Input: part model. Units: mm. Frame: model coordinates. Round coordinates to 2 decimals unless told otherwise and drop trailing zeros. Loops run counter-clockwise (first coordinate to the right, second up) from the corner with the lowest first, then second, coordinate; pieces in that order, holes last. Notation, with made-up numbers: M 66.25,-30 L 112.25,-30 A21 cw 112.25,-24 Z; hole C 35.25,19 d8. An arc over 180 degrees is marked long. Use one line per item in the form item = value. Start each with the question number.
Q1. Section query D-D, the plane x = 173. Output: boundary loops of the cut face in (y, z), and give its area (3 significant figures).
Q2. First-contact query: P1, Ø2, axis at x = 38, y = 2, coming from the -Z side; P2, Ø1.5, axis at x = 132.5, y = 3.5, coming from the +Z side; P3, Ø2.5, axis at y = 2.5, z = -45, coming from the -X side. Flat tips, straight axial feed; report the tip coordinate or a pass-through.
Q3. Section query A-A, the plane x = 25. Output: boundary loops of the cut face in (y, z), and give its area (3 significant figures).
Q4. Ray query, line 1 along X through (y, z) = (0.7, 62.5); line 2 along Z through (x, y) = (108, 2.55); line 3 along Z through (x, y) = (184, 3.8). Return the intervals inside material, ascending.
Q5. Section query B-B, the plane y = 2.2. State how many separate pieces and enclosed holes the cut face has, and give its area (3 significant figures).
Q6. Section query C-C, the plane z = 153. Output: boundary loops of the cut face in (x, y).
```python
from build123d import *

# Parameters (mm, degrees)
SKETCH1_W           = 220
SKETCH1_H           = 160
SKETCH1_W_2         = 160
SKETCH1_H_2         = 100
SKETCH1_W_3         = 73
SKETCH1_H_3         = 14
SKETCH1_W_4         = 14
SKETCH1_H_4         = 43
BOSS_EXTRUDE1_DEPTH = 5
SKETCH2_R           = 1.5
CUT_EXTRUDE1_DEPTH  = 5
SKETCH3_W           = 14
SKETCH3_H           = 60
BOSS_EXTRUDE2_DEPTH = 5


with BuildPart() as part:
    # Sketch1 → Boss-Extrude1 (new body)
    # profile 1 of 6: a face of its own
    with BuildSketch(Plane(origin=(0, 0, 0), x_dir=(1, 0, 0), z_dir=(0, 1, 0))):
        with Locations((80, -50)):
            Rectangle(SKETCH1_W, SKETCH1_H)
        with Locations((80, -50)):
            Rectangle(SKETCH1_W_2, SKETCH1_H_2, mode=Mode.SUBTRACT)
    # profile 2 of 6: a face of its own
    with BuildSketch(Plane(origin=(0, 0, 0), x_dir=(1, 0, 0), z_dir=(0, 1, 0))):
        with Locations((36.5, -50)):
            Rectangle(SKETCH1_W_3, SKETCH1_H_3)
    # profile 3 of 6: a face of its own
    with BuildSketch(Plane(origin=(0, 0, 0), x_dir=(1, 0, 0), z_dir=(0, 1, 0))):
        with Locations((123.5, -50)):
            Rectangle(SKETCH1_W_3, SKETCH1_H_3)
    # profile 4 of 6: a face of its own
    with BuildSketch(Plane(origin=(0, 0, 0), x_dir=(1, 0, 0), z_dir=(0, 1, 0))):
        with Locations((80, -21.5)):
            Rectangle(SKETCH1_W_4, SKETCH1_H_4)
    # profile 5 of 6: a face of its own
    with BuildSketch(Plane(origin=(0, 0, 0), x_dir=(1, 0, 0), z_dir=(0, 1, 0))):
        with Locations((80, -78.5)):
            Rectangle(SKETCH1_W_4, SKETCH1_H_4)
    # profile 6 of 6: a face of its own
    with BuildSketch(Plane(origin=(0, 0, 0), x_dir=(1, 0, 0), z_dir=(0, 1, 0))):
        with Locations((80, -50)):
            Rectangle(SKETCH1_W_4, SKETCH1_H_3)
    extrude(amount=BOSS_EXTRUDE1_DEPTH)

    # Sketch2 → Cut-Extrude1 (cut)
    with BuildSketch(Plane(origin=(0, 5, 0), x_dir=(1, 0, 0), z_dir=(0, 1, 0))):
        with Locations(Location((-24, -29, 0), (0, 0, 270))):
            Circle(SKETCH2_R)
        with Locations(Location((-24, -71, 0), (0, 0, 90))):
            Circle(SKETCH2_R)
        with Locations(Location((184, -29, 0), (0, 0, 90))):
            Circle(SKETCH2_R)
        with Locations(Location((184, -71, 0), (0, 0, 270))):
            Circle(SKETCH2_R)
    extrude(amount=-CUT_EXTRUDE1_DEPTH, mode=Mode.SUBTRACT)

    # Sketch3 → Boss-Extrude2 (add)
    with BuildSketch(Plane(origin=(0, 5, 0), x_dir=(1, 0, 0), z_dir=(0, 1, 0))):
        with Locations((80, 60)):
            Rectangle(SKETCH3_W, SKETCH3_H)
        with Locations((80, -160)):
            Rectangle(SKETCH3_W, SKETCH3_H)
    extrude(amount=-BOSS_EXTRUDE2_DEPTH)


solid = part.part
```
Results found:
q1.outline = M 0,-30 L 5,-30 L 5,130 L 0,130 Z
q1.area = 800 mm²
q2.P1 = -30
q2.P2 = 130
q2.P3 = 73
q3.outline = M 0,-30 L 5,-30 L 5,0 L 0,0 Z; M 0,43 L 5,43 L 5,57 L 0,57 Z; M 0,100 L 5,100 L 5,130 L 0,130 Z
q3.area = 370 mm²
q4.line_1 = -30 to 0, 73 to 87, 160 to 190
q4.line_2 = -30 to 0, 43 to 57, 100 to 130
q4.line_3 = -30 to 27.5, 30.5 to 69.5, 72.5 to 130
q5.separate_pieces = 1
q5.enclosed_holes = 8
q5.area = 24,300 mm²
q6.outline = M 73,0 L 87,0 L 87,5 L 73,5 Z
